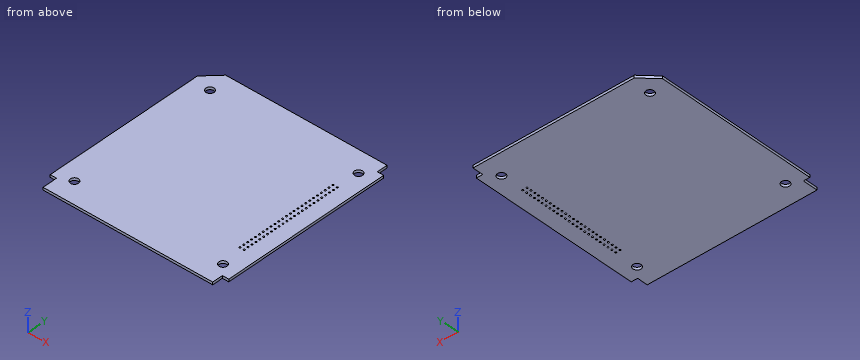
```python
from build123d import *

# Parameters (mm, degrees)
SKETCH1_R           = 1.9
SKETCH1_R_2         = 0.375
SKETCH1_R_3         = 0.383755901
SKETCH1_R_4         = 0.384163196
SKETCH1_R_5         = 0.380771211
SKETCH1_R_6         = 0.377379225
SKETCH1_R_7         = 0.380832793
BOSS_EXTRUDE1_DEPTH = 1.2
SKETCH_1_W          = 3
SKETCH_1_H          = 7
CUT_EXTRUDE_1_DEPTH = 10


with BuildPart() as part:
    # Sketch1 → Boss-Extrude1 (new body)
    with BuildSketch(Plane.XY):
        Polygon((-3, 0), (-86, 0), (-86, -90), (-3, -90), (-3, -85), (0, -85), (0, -5), (-3, -5), align=None)
        with Locations((-7.3, -10)):
            Circle(SKETCH1_R, mode=Mode.SUBTRACT)
        with Locations((-77.3, -10)):
            Circle(SKETCH1_R, mode=Mode.SUBTRACT)
        with Locations((-77.3, -80)):
            Circle(SKETCH1_R, mode=Mode.SUBTRACT)
        with Locations((-7.3, -80)):
            Circle(SKETCH1_R, mode=Mode.SUBTRACT)
        with Locations((-9.3, -69)):
            Circle(SKETCH1_R_2, mode=Mode.SUBTRACT)
        with Locations((-7.3, -69)):
            Circle(SKETCH1_R_2, mode=Mode.SUBTRACT)
        with Locations((-7.3, -67)):
            Circle(SKETCH1_R_2, mode=Mode.SUBTRACT)
        with Locations((-9.3, -67)):
            Circle(SKETCH1_R_2, mode=Mode.SUBTRACT)
        with Locations((-9.3, -65)):
            Circle(SKETCH1_R_2, mode=Mode.SUBTRACT)
        with Locations((-7.3, -65)):
            Circle(SKETCH1_R_2, mode=Mode.SUBTRACT)
        with Locations((-7.3, -63)):
            Circle(SKETCH1_R_2, mode=Mode.SUBTRACT)
        with Locations((-9.3, -63)):
            Circle(SKETCH1_R_3, mode=Mode.SUBTRACT)
        with Locations((-9.3, -61)):
            Circle(SKETCH1_R_2, mode=Mode.SUBTRACT)
        with Locations((-7.3, -61)):
            Circle(SKETCH1_R_2, mode=Mode.SUBTRACT)
        with Locations((-7.3, -59)):
            Circle(SKETCH1_R_2, mode=Mode.SUBTRACT)
        with Locations((-9.3, -59)):
            Circle(SKETCH1_R_2, mode=Mode.SUBTRACT)
        with Locations((-7.3, -57)):
            Circle(SKETCH1_R_2, mode=Mode.SUBTRACT)
        with Locations((-9.3, -57)):
            Circle(SKETCH1_R_2, mode=Mode.SUBTRACT)
        with Locations((-9.3, -55)):
            Circle(SKETCH1_R_2, mode=Mode.SUBTRACT)
        with Locations((-7.3, -55)):
            Circle(SKETCH1_R_2, mode=Mode.SUBTRACT)
        with Locations((-7.3, -53)):
            Circle(SKETCH1_R_2, mode=Mode.SUBTRACT)
        with Locations((-9.3, -53)):
            Circle(SKETCH1_R_2, mode=Mode.SUBTRACT)
        with Locations((-9.3, -51)):
            Circle(SKETCH1_R_2, mode=Mode.SUBTRACT)
        with Locations((-7.3, -51)):
            Circle(SKETCH1_R_2, mode=Mode.SUBTRACT)
        with Locations((-7.3, -49)):
            Circle(SKETCH1_R_2, mode=Mode.SUBTRACT)
        with Locations((-9.3, -49)):
            Circle(SKETCH1_R_2, mode=Mode.SUBTRACT)
        with Locations((-9.3, -47)):
            Circle(SKETCH1_R_2, mode=Mode.SUBTRACT)
        with Locations((-7.3, -47)):
            Circle(SKETCH1_R_2, mode=Mode.SUBTRACT)
        with Locations((-7.3, -45)):
            Circle(SKETCH1_R_2, mode=Mode.SUBTRACT)
        with Locations((-9.3, -45)):
            Circle(SKETCH1_R_4, mode=Mode.SUBTRACT)
        with Locations((-9.3, -43)):
            Circle(SKETCH1_R_2, mode=Mode.SUBTRACT)
        with Locations((-7.3, -43)):
            Circle(SKETCH1_R_5, mode=Mode.SUBTRACT)
        with Locations((-7.3, -41)):
            Circle(SKETCH1_R_6, mode=Mode.SUBTRACT)
        with Locations((-9.3, -41)):
            Circle(SKETCH1_R_6, mode=Mode.SUBTRACT)
        with Locations((-9.3, -39)):
            Circle(SKETCH1_R_2, mode=Mode.SUBTRACT)
        with Locations((-7.3, -39)):
            Circle(SKETCH1_R_2, mode=Mode.SUBTRACT)
        with Locations((-7.3, -37)):
            Circle(SKETCH1_R_2, mode=Mode.SUBTRACT)
        with Locations((-9.3, -37)):
            Circle(SKETCH1_R_7, mode=Mode.SUBTRACT)
        with Locations((-7.3, -35)):
            Circle(SKETCH1_R_2, mode=Mode.SUBTRACT)
        with Locations((-9.3, -35)):
            Circle(SKETCH1_R_2, mode=Mode.SUBTRACT)
        with Locations((-9.3, -33)):
            Circle(SKETCH1_R_2, mode=Mode.SUBTRACT)
        with Locations((-7.3, -33)):
            Circle(SKETCH1_R_2, mode=Mode.SUBTRACT)
        with Locations((-7.3, -31)):
            Circle(SKETCH1_R_2, mode=Mode.SUBTRACT)
        with Locations((-9.3, -31)):
            Circle(SKETCH1_R_2, mode=Mode.SUBTRACT)
        with Locations((-7.3, -29)):
            Circle(SKETCH1_R_2, mode=Mode.SUBTRACT)
        with Locations((-9.3, -29)):
            Circle(SKETCH1_R_2, mode=Mode.SUBTRACT)
        with Locations((-9.3, -27)):
            Circle(SKETCH1_R_2, mode=Mode.SUBTRACT)
        with Locations((-7.3, -27)):
            Circle(SKETCH1_R_2, mode=Mode.SUBTRACT)
        with Locations((-7.3, -25)):
            Circle(SKETCH1_R_2, mode=Mode.SUBTRACT)
        with Locations((-9.3, -25)):
            Circle(SKETCH1_R_2, mode=Mode.SUBTRACT)
        with Locations((-7.3, -23)):
            Circle(SKETCH1_R_2, mode=Mode.SUBTRACT)
        with Locations((-9.3, -23)):
            Circle(SKETCH1_R_2, mode=Mode.SUBTRACT)
        with Locations((-9.3, -21)):
            Circle(SKETCH1_R_2, mode=Mode.SUBTRACT)
        with Locations((-7.3, -21)):
            Circle(SKETCH1_R_2, mode=Mode.SUBTRACT)
    extrude(amount=BOSS_EXTRUDE1_DEPTH)

    # ｽｹｯﾁ1 → ｶｯﾄ - 押し出し1 (cut)
    with BuildSketch(Plane.XY.offset(1.2)):
        with Locations((-84.5, -86.5)):
            Rectangle(SKETCH_1_W, SKETCH_1_H)
        Polygon((-86, -7), (-86, 0), (-79, 0), align=None)
    extrude(amount=-CUT_EXTRUDE_1_DEPTH, mode=Mode.SUBTRACT)


solid = part.part
```
CAD build for the part. Positions are in the model's coordinates, mm. Round coordinates to 2 decimals unless told otherwise and drop trailing zeros. Loops run counter-clockwise (first coordinate to the right, second up) from the corner with the lowest first, then second, coordinate; pieces in that order, holes last. Notation, with made-up numbers: M 78,83.25 L 113,83.25 A29 ccw 113,106.25 Z; hole C 80.5,-32 d3. An arc over 180 degrees is marked long. Use a Markdown table: item, result. Add a question column.
(1) Flat gauge pin, fed straight in: pin 1 (3 mm diameter, centred on x = -77.3, y = -80, fed in from -Z) (3 decimals). Where does the tip first touch, or does it go through?
(2) Cut at A-A (x = -77.3). Give the cut face in (y, z).
(3) Cut at B-B (z = 0.25). State how many separate pieces and enclosed holes the cut face has, and give its area (3 significant figures).
(4) Drill centre lines: line 1 (X direction, y = -67, z = 0.8) (3 decimals); line 2 (X direction, y = -9, z = 0.1); line 3 (Y direction, x = -78, z = 0.3). Where is each one in solid material? Low to high.
Geometry says:
| question | item | result |
|---|---|---|
| 1 | pin 1 | passes through |
| 2 | outline | M -90,0 L -81.9,0 L -81.9,1.2 L -90,1.2 Z; M -78.1,0 L -11.9,0 L -11.9,1.2 L -78.1,1.2 Z; M -8.1,0 L 0,0 L 0,1.2 L -8.1,1.2 Z |
| 3 | separate pieces | 1 |
| 3 | enclosed holes | 54 |
| 3 | area | 7,600 mm² |
| 4 | line 1 | x = -86 to -9.675, -8.925 to -7.675, -6.925 to 0 |
| 4 | line 2 | x = -86 to -78.92, -75.68 to -8.92, -5.68 to 0 |
| 4 | line 3 | y = -90 to -81.77, -78.23 to -11.77, -8.23 to 0 |
